Check sheet for the modelled part. Datum: model origin and axes. Units: mm. A direction names the side the tool comes from. Round coordinates to 2 decimals unless told otherwise and drop trailing zeros. Loops run counter-clockwise (first coordinate to the right, second up) from the corner with the lowest first, then second, coordinate; pieces in that order, holes last. Notation, with made-up numbers: (-13, 48.25) -> (7, 48.25) arc R20 cw to (7, 79.25) -> close; hole circle Ø1 at (7, -3.75). An arc over 180 degrees is marked (long way). Use one line per item in the form item = value. Start each with the question number.
(1) Sectioned sample at D-D (y = 5.25). Record the cut outline in (x, z).
(2) Sectioned sample at A-A (y = 11.5). Record the cut outline in (x, z) (3 decimals).
(3) Go/stop test with flat-tipped pins: pin 1 (3 mm diameter, centred on x = -1, z = 2, fed in from -Y); pin 2 (1.4 mm diameter, centred on y = 6, z = 0, fed in from +X); pin 3 (2 mm diameter, centred on y = 5.5, z = 0.5, fed in from -X); pin 4 (3 mm diameter, centred on x = 0, y = 3, fed in from +Z). Record where each tip stops, or that it passes through.
(4) Set-up check for faces 1 (the flat face through (1.388, 5, 0)), 2 (the flat face through (-1.388, 5, 0)), 3 (the flat face through (0, 5, -1.388)), 4 (the flat face through (0, 10.775, -3)), 5 (the flat face through (0, 5, 1.388)): record each of +Z, -Z, +X, -X, +Y, -Y from which the full face is reachable in a straight line by a thin tool's end or side.
(5) Material ranges on probe 1 along Y at (x, z) = (-0.5, 2.75) (3 decimals); probe 2 along Z at (x, y) = (-1, 4.75), recorded low to high. Write a range as [from, to].
from build123d import *

# Parameters (mm, degrees)
SKETCH1_W           = 2.775
SKETCH1_H           = 2.775
BOSS_EXTRUDE1_DEPTH = 10.775
SKETCH2_W           = 6.35
SKETCH2_H           = 7.9375
BOSS_EXTRUDE2_DEPTH = 3.175
FILLET1_R           = 1.25


with BuildPart() as part:
    # Sketch1 → Boss-Extrude1 (new body)
    with BuildSketch(Plane(origin=(0, 0, 0), x_dir=(1, 0, 0), z_dir=(0, 1, 0))):
        Rectangle(SKETCH1_W, SKETCH1_H)
    extrude(amount=BOSS_EXTRUDE1_DEPTH)

    # Sketch2 → Boss-Extrude2 (add)
    with BuildSketch(Plane(origin=(0, 10.775, 0), x_dir=(1, 0, 0), z_dir=(0, 1, 0))):
        Rectangle(SKETCH2_W, SKETCH2_H)
    extrude(amount=BOSS_EXTRUDE2_DEPTH)

    # Fillet1
    fillet1_edges = [part.edges().sort_by_distance(p)[0] for p in [
        (-1.3875, 10.775, 0),
        (0, 10.775, 1.3875),
        (1.3875, 10.775, 0),
        (0, 10.775, -1.3875),
    ]]
    fillet(fillet1_edges, radius=FILLET1_R)
    fillet1_2_edges = [part.edges().sort_by_distance(p)[0] for p in [
        (3.175, 12.3625, 3.96875),
        (3.175, 12.3625, -3.96875),
        (-3.175, 12.3625, -3.96875),
        (-3.175, 12.3625, 3.96875),
    ]]
    fillet(fillet1_2_edges, radius=FILLET1_R)


solid = part.part
Checks:
q1.outline = (-1.39, -1.39) -> (1.39, -1.39) -> (1.39, 1.39) -> (-1.39, 1.39) -> close
q2.outline = (-3.175, -2.719) arc R1.25 ccw to (-1.925, -3.969) -> (1.925, -3.969) arc R1.25 ccw to (3.175, -2.719) -> (3.175, 2.719) arc R1.25 ccw to (1.925, 3.969) -> (-1.925, 3.969) arc R1.25 ccw to (-3.175, 2.719) -> close
q3.pin_1 = 0
q3.pin_2 = 1.39
q3.pin_3 = -1.39
q3.pin_4 = 1.39
q4.face_1 = +Z, -Z, +X, -Y
q4.face_2 = +Z, -Z, -X, -Y
q4.face_3 = -Z, +X, -X, -Y
q4.face_4 = -Y
q4.face_5 = +Z, +X, -X, -Y
q5.probe_1 = [10.775, 13.95]
q5.probe_2 = [-1.39, 1.39]
